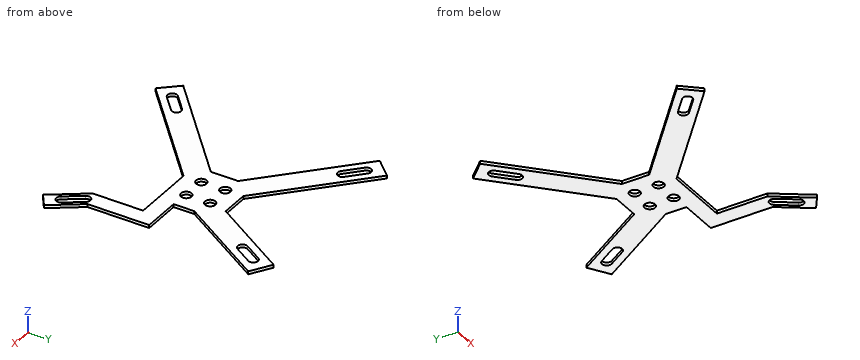
Autodesk Inventor part; units mm, degrees
ref_plane "YZ Plane" through (0, 0, 0) normal (1, 0, 0) x (0, 1, 0)
ref_plane "XZ Plane" through (0, 0, 0) normal (0, 1, 0) x (-1, 0, 0)
ref_plane "XY Plane" through (0, 0, 0) normal (0, 0, 1) x (1, 0, 0)
sketch "Sketch1" plane through (0, 0, 0) normal (0, 0, 1) x (1, 0, 0)
  line L0 (-10, 10) -> (10, 10)
  line L1 (10, 10) -> (10, -10)
  line L2 (10, -10) -> (-10, -10)
  line L3 (-10, -10) -> (-10, 10)
  line L4 (-10, 10) -> (10, -10) construction
  line L5 (10, 10) -> (-10, -10) construction
  circle A0 centre (-4, 4) radius 1.75
  line L6 (-4, 4) -> (0.2191, 4)
  line L7 (0.2191, 4) -> (0.2191, 2.6146)
  circle A1 centre (4, 4) radius 1.75
  circle A2 centre (-4, -4) radius 1.75
  circle A3 centre (4, -4) radius 1.75
  point P0 (0, 0)
  dimension "d0" = 20
  dimension "d1" = 20
  dimension "d2" = 3.5
  dimension "d5" = 8
  dimension "d8" = 8
  dimension "d11" = 4
  dimension "d12" = 4
extrude "Plate1" add sketch "Sketch1" along normal blind 1
sketch "Sketch2" plane through (0, 0, 1) normal (0, 0, 1) x (1, 0, 0)
  line L0 (-10, -10) -> (-10, 10)
  line L1 (-10, 10) -> (-33.9394, 32.3238)
  line L2 (-10, -10) -> (-37.6112, -34.8612)
  line L3 (-10, 10) -> (10, 10)
  line L4 (10, 10) -> (17.9255, 22.6834)
  line L5 (10, -10) -> (-10, -10)
  line L6 (-40.4218, 32.8995) -> (-8.9736, 3.5735)
  line L7 (-8.9736, 3.5735) -> (-3.5176, 9.4244)
  line L8 (-3.5176, 9.4244) -> (-34.9658, 38.7503)
  line L9 (-34.9658, 38.7503) -> (-40.4218, 32.8995)
  line L10 (-40.4218, 32.8995) -> (-3.5176, 9.4244) construction
  line L11 (-8.9736, 3.5735) -> (-34.9658, 38.7503) construction
  line L12 (10, 10) -> (10, -10)
  line L13 (-44.0946, -35.3164) -> (-8.8696, -3.5996)
  line L14 (-8.8696, -3.5996) -> (-3.5165, -9.5448)
  line L15 (-3.5165, -9.5448) -> (-38.7416, -41.2616)
  line L16 (-38.7416, -41.2616) -> (-44.0946, -35.3164)
  line L17 (-44.0946, -35.3164) -> (-3.5165, -9.5448) construction
  line L18 (-8.8696, -3.5996) -> (-38.7416, -41.2616) construction
  line L19 (28.6116, 32.2365) -> (9.9585, 2.3852)
  line L20 (9.9585, 2.3852) -> (3.1741, 6.6246)
  line L21 (3.1741, 6.6246) -> (21.8273, 36.4759)
  line L22 (21.8273, 36.4759) -> (28.6116, 32.2365)
  line L23 (28.6116, 32.2365) -> (3.1741, 6.6246) construction
  line L24 (9.9585, 2.3852) -> (21.8273, 36.4759) construction
  line L25 (23, -4.5) -> (10, -4.5)
  line L26 (10, -4.5) -> (10, -10)
  line L27 (10, -10) -> (23, -10)
  line L28 (23, -10) -> (23, -4.5)
  line L29 (23, -4.5) -> (10, -10) construction
  line L30 (10, -4.5) -> (23, -10) construction
  line L31 (17.5, -26.9397) -> (17.5, -10)
  line L32 (17.5, -10) -> (23, -10)
  line L33 (23, -10) -> (23, -30)
  line L34 (23, -30) -> (19.6429, -30)
  line L35 (16.1337, -34.9685) -> (23, -10) construction
  line L36 (17.5, -10) -> (23, -30) construction
  line L37 (25.5844, -38.4854) -> (17.5, -26.9397)
  line L38 (17.5, -26.9397) -> (22.0053, -23.785)
  line L39 (22.0053, -23.785) -> (30.0897, -35.3307)
  line L40 (30.0897, -35.3307) -> (25.5844, -38.4854)
  line L41 (25.5844, -38.4854) -> (22.0053, -23.785) construction
  line L42 (17.5, -26.9397) -> (30.0897, -35.3307) construction
  line L43 (23, -30) -> (23.7949, -31.1352)
  point P0 (0, 0)
  point P1 (-21.9697, 21.1619)
  point P2 (-23.8056, -22.4306)
  point P3 (15.8929, 19.4306)
  point P4 (16.5, -7.25)
  point P5 (20.25, -20)
  dimension "d14" = 137
  dimension "d15" = 138
  dimension "d17" = 148
  dimension "d18" = 8
  dimension "d19" = 8
  dimension "d21" = 8
  dimension "d22" = 42.5
  dimension "d23" = 7.3
  dimension "d24" = 9
  dimension "d25" = 9
  dimension "d28" = 56.4
  dimension "d29" = 52
  dimension "d35" = 5.5
  dimension "d36" = 5.5
  dimension "d38" = 13
  dimension "d39" = 20
  dimension "d41" = 5.5
  dimension "d42" = 145
  dimension "d43" = 46.2
sheet face with bend "Face2" sketch "Sketch2" thickness 1 toward (0, 0, -1) bend radius 1 contours L5 L15 L16 L13 L0 | L0 L13 L14 L15 L5 | L6 L9 L8 L3 L0 | L0 L3 L8 L7 L6 | L12 L25 L28 L27 | L27 L33 L39 L38 L31 | L19 L20 L21 L3 L12 | L12 L3 L21 L22 L19 | L38 L39 L33 L34 L37 | L39 L40 L37 L34 L33
bend "Bend1"
sketch "Sketch4" plane through (0, 0, 1) normal (0, 0, 1) x (1, 0, 0)
  circle A0 centre (-32.5004, -30.2594) radius 1.6
  circle A1 centre (-37.7024, -34.9433) radius 1.6
  circle A2 centre (-34.037, 32.4149) radius 1.6
  circle A3 centre (-28.9175, 27.6409) radius 1.6
  circle A4 centre (22.5699, 30.116) radius 1.6
  circle A5 centre (18.8604, 24.1796) radius 1.6
  line L0 (-34.037, 32.4149) -> (-28.9175, 27.6409)
  line L1 (22.5699, 30.116) -> (18.8604, 24.1796)
  line L2 (-37.7024, -34.9433) -> (-32.5004, -30.2594)
  line L3 (20.9542, -27.0782) -> (24.9692, -32.8123)
  line L4 (30.0897, -35.3307) -> (23, -25.2055)
  circle A6 centre (20.9542, -27.0782) radius 1.6
  circle A7 centre (24.9692, -32.8123) radius 1.6
  line L5 (25.5844, -38.4854) -> (30.0897, -35.3307)
  line L6 (28.6116, 32.2365) -> (10, 2.4517)
  line L7 (-4.1349, 10) -> (-34.9658, 38.7503)
  line L8 (-44.0946, -35.3164) -> (-10, -4.6175)
  line L9 (-38.7416, -41.2616) -> (-44.0946, -35.3164)
  line L10 (21.8273, 36.4759) -> (28.6116, 32.2365)
  line L11 (-34.9658, 38.7503) -> (-40.4218, 32.8995)
  line L12 (-37.7024, -34.9433) -> (-32.5004, -30.2594) construction
  line L13 (-36.6318, -36.1324) -> (-31.4298, -31.4485)
  line L14 (-33.571, -29.0704) -> (-38.773, -33.7543)
  arc A8 (-38.773, -33.7543) -> (-36.6318, -36.1324) centre (-37.7024, -34.9433) ccw
  arc A9 (-31.4298, -31.4485) -> (-33.571, -29.0704) centre (-32.5004, -30.2594) ccw
  line L15 (20.9542, -27.0782) -> (24.9692, -32.8123) construction
  line L16 (19.6435, -27.996) -> (23.6585, -33.73)
  line L17 (26.2798, -31.8946) -> (22.2648, -26.1605)
  arc A10 (22.2648, -26.1605) -> (19.6435, -27.996) centre (20.9542, -27.0782) ccw
  arc A11 (23.6585, -33.73) -> (26.2798, -31.8946) centre (24.9692, -32.8123) ccw
  line L18 (18.8604, 24.1796) -> (22.5699, 30.116) construction
  line L19 (20.2173, 23.3318) -> (23.9267, 29.2681)
  line L20 (21.213, 30.9638) -> (17.5035, 25.0275)
  arc A12 (17.5035, 25.0275) -> (20.2173, 23.3318) centre (18.8604, 24.1796) ccw
  arc A13 (23.9267, 29.2681) -> (21.213, 30.9638) centre (22.5699, 30.116) ccw
  line L21 (-28.9175, 27.6409) -> (-34.037, 32.4149) construction
  line L22 (-27.8263, 28.8111) -> (-32.9458, 33.5851)
  line L23 (-35.1282, 31.2447) -> (-30.0087, 26.4707)
  arc A14 (-30.0087, 26.4707) -> (-27.8263, 28.8111) centre (-28.9175, 27.6409) ccw
  arc A15 (-32.9458, 33.5851) -> (-35.1282, 31.2447) centre (-34.037, 32.4149) ccw
  point P0 (0, 0)
  point P1 (-35.1014, -32.6014)
  point P2 (22.9617, -29.9453)
  point P3 (20.7151, 27.1478)
  point P4 (-31.4773, 30.0279)
  dimension "d54" = 2.75
  dimension "d55" = 3.2
  dimension "d56" = 3.2
  dimension "d58" = 5
  dimension "d59" = 7
  dimension "d60" = 3.2
  dimension "d61" = 3.2
  dimension "d62" = 3.2
  dimension "d63" = 3.2
  dimension "d64" = 3.2
  dimension "d65" = 3.2
  dimension "d66" = 8
  dimension "d67" = 8
  dimension "d68" = 8
  dimension "d69" = 5
  dimension "d70" = 7
  dimension "d71" = 5
  dimension "d72" = 7
  dimension "d73" = 5
  dimension "d74" = 7
extrude "Cut1" cut sketch "Sketch4" against normal blind 1
sketch "Sketch3" plane through (-41.7142, -43.9381, 0) normal (-0.7431448, -0.6691306, 0) x (0.6691306, -0.7431448, 0)
  line L0 (-8, 0) -> (0, 0)
  line L1 (0, 0) -> (0, 25)
  line L2 (0, 25) -> (-8, 25)
  line L3 (-8, 25) -> (-8, 0)
equation "\"d75\" = 厚度"
equation "\"d13\" = 厚度"
equation "\"d30\" = 折彎半徑"
equation "\"d31\" = 折彎離隙寬度"
equation "\"d33\" = 最小剩餘"
equation "\"d32\" = 折彎離隙深度"
equation "\"d34\" = 轉移半徑"
equation "\"折彎半徑\" = 厚度"
equation "\"折彎離隙寬度\" = 厚度"
equation "\"折彎離隙深度\" = 0.5 * 厚度"
equation "\"轉角離隙大小\" = 4 * 厚度"
equation "\"最小剩餘\" = 2 * 厚度"
equation "\"轉移半徑\" = 折彎半徑"
equation "\"Jacobi半徑大小\" = 折彎半徑"
equation "\"間隙大小\" = 厚度"
properties part number "watercooler_fixed2"
Could you check a few things on this model? Use its own coordinates, in mm. Coordinates: 2 decimals unless noted, no trailing zeros. Loops run counter-clockwise (first coordinate to the right, second up) from the corner with the lowest first, then second, coordinate; pieces in that order, holes last.
1. Imagine slicing it at C-C (y = -18). Please give me the cut outline in (x, z).
2. Imagine slicing it at B-B (x = -16). Please give me the cut outline in (y, z), and give its area (3 significant figures).
3. I need wall thicknesses on L1, parallel to Y at x = 4, z = 0.85; L2, parallel to X at y = 5, z = 0.95; L3, parallel to Y at x = -4.5, z = 0.7. Which ranges of each line are inside material? Lowest first, please.
4. Imagine slicing it at A-A (x = 4). Please give me the cut outline in (y, z).
5. Imagine slicing it at D-D (z = 0.4). Give the number of separate pieces and of enclosed holes in the cut face, and give its area (3 significant figures).
6. For P1, Ø3, axis at x = -4, y = 4, coming from the +Z side, with a flat end and sliding along its axis, tell me the tip position at first contact or that it passes through.
Computed values:
1. outline: (-24.86, 0) - (-12.91, 0) - (-12.91, 1) - (-24.86, 1) - close; (17.5, 0) - (23, 0) - (23, 1) - (17.5, 1) - close
2. outline: (-20.78, 0) - (-10.02, 0) - (-10.02, 1) - (-20.78, 1) - close; (10.13, 0) - (21.06, 0) - (21.06, 1) - (10.13, 1) - close
2. area: 21.7 mm2
3. L1: y = -10 to -5.75, -2.25 to 2.25, 5.75 to 10
3. L2: x = -10.5 to -5.44, -2.56 to 2.56, 5.44 to 11.59
3. L3: y = -10.43 to -5.68, -2.32 to 2.32, 5.68 to 10.34
4. outline: (-10, 0) - (-5.75, 0) - (-5.75, 1) - (-10, 1) - close; (-2.25, 0) - (2.25, 0) - (2.25, 1) - (-2.25, 1) - close; (5.75, 0) - (10, 0) - (10, 1) - (5.75, 1) - close
5. separate pieces: 1
5. enclosed holes: 8
5. area: 1,390 mm2
6. P1: passes through
